Model file for the job. Use its own axes, mm. Face numbers are marked on the shaded views. A direction names the side the tool comes from. Coordinates: 2 decimals unless noted, no trailing zeros. Order: outer loops, then holes, each group sorted by start corner. A loop starts at its lowest first (then second) coordinate and runs counter-clockwise, first axis right, second up. Notation, with made-up numbers: (34.25, 34) -> (62.25, 34) arc R32 cw to (62.25, 64) -> close; hole circle Ø10 at (85.5, 39). An arc over 180 degrees is marked (long way). Use CSV: the item, a comma, the result in double quotes. Start each with the question number.
(1) Pin check, flat tips, straight feed: pin 1 Ø0.9 at (x, y) = (1.5, -11) entering from +Z; pin 2 Ø0.9 at (x, y) = (1.5, -7) entering from +Z; pin 3 Ø0.9 at (x, z) = (1.5, -21) entering from +Y. Stop position of each tip, or through.
(2) Pull direction Z, two halves, no side cores. Call the marked faces 1, 2, 3 and 4: pulls with the +Z half, pulls with the -Z half, needs draft (parallel to the pull), parting line crosses it, or undercut.
(3) Cut at D-D on y = 6.5. Write the cut outline in (x, z), plus the area to 3 significant figures.
(4) Tool access for the marked faces 5, 6 and 7: list every direction of +Z, -Z, +X, -X, +Y, -Y with a clear straight run to the whole face (end or side of a thin tool).
(5) Cut at B-B on x = 2.55. Write the cut outline in (y, z), plus the area to 3 significant figures.
(6) Cut at C-C on z = -1. Write the cut outline in (x, y).
(7) Probe L1, parallel to Z at x = 2.7, y = -9.5; L2, parallel to Z at x = 2, y = 8.75; L3, parallel to Y at x = 2.4, z = -18.5. List the from-to ranges inside material, lowest first.
(8) Cut at A-A on y = -10. Write the cut outline in (x, z).
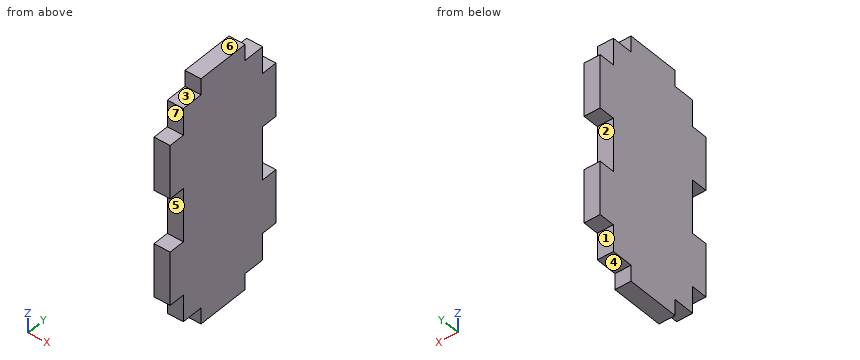
```python
from build123d import *

# Parameters (mm, degrees)
SKETCH1_W               = 46
SKETCH1_H               = 24
BOSS_EXTRUDE1_DEPTH     = 3
SKETCH2_W               = 5
SKETCH2_H               = 3
CUT_EXTRUDE1_DEPTH      = 4
MIRROR2_COPY_1_SKETCH_W = 5
MIRROR2_COPY_1_SKETCH_H = 3
MIRROR2_COPY_1_DEPTH    = 4


with BuildPart() as part:
    # Sketch1 → Boss-Extrude1 (new body)
    with BuildSketch(Plane(origin=(0, 0, 0), x_dir=(0, 0, -1), z_dir=(1, 0, 0))):
        Rectangle(SKETCH1_W, SKETCH1_H)
    extrude(amount=BOSS_EXTRUDE1_DEPTH)

    # Sketch2 → Cut-Extrude1 (cut, through all)
    with BuildSketch(Plane(origin=(3, 0, 0), x_dir=(0, 0, -1), z_dir=(1, 0, 0))):
        Polygon((23, 5), (20, 5), (20, 9), (15, 9), (15, 12), (23, 12), align=None)
        with Locations((2.5, 10.5)):
            Rectangle(SKETCH2_W, SKETCH2_H)
    cut_extrude1 = extrude(amount=-CUT_EXTRUDE1_DEPTH, mode=Mode.SUBTRACT)

    # Mirror1: Cut-Extrude1 across plane
    add(cut_extrude1.mirror(Plane.ZX), mode=Mode.SUBTRACT)

    # Mirror2: Cut-Extrude1 across plane
    add(cut_extrude1.mirror(Plane.XY), mode=Mode.SUBTRACT)

    # Mirror2 copy 1 sketch → Mirror2 copy 1 (cut, through all)
    with BuildSketch(Plane(origin=(3, 0, 0), x_dir=(0, 0, 1), z_dir=(1, 0, 0))):
        Polygon((23, 5), (20, 5), (20, 9), (15, 9), (15, 12), (23, 12), align=None)
        with Locations((2.5, 10.5)):
            Rectangle(MIRROR2_COPY_1_SKETCH_W, MIRROR2_COPY_1_SKETCH_H)
    extrude(amount=-MIRROR2_COPY_1_DEPTH, mode=Mode.SUBTRACT)


solid = part.part
```
Outcome:
1,pin 1,"z = 15"
1,pin 2,"z = 20"
1,pin 3,"y = 5"
2,face 1,"needs draft"
2,face 2,"undercut"
2,face 3,"pulls with the +Z half"
2,face 4,"pulls with the -Z half"
3,outline,"(0, -20) -> (3, -20) -> (3, 20) -> (0, 20) -> close"
3,area,"120 mm2"
4,face 5,"+X, -X, -Y"
4,face 6,"+Z, +X, -X, +Y, -Y"
4,face 7,"+Z, +X, -X, -Y"
5,outline,"(-12, -15) -> (-9, -15) -> (-9, -20) -> (-5, -20) -> (-5, -23) -> (5, -23) -> (5, -20) -> (9, -20) -> (9, -15) -> (12, -15) -> (12, -5) -> (9, -5) -> (9, 5) -> (12, 5) -> (12, 15) -> (9, 15) -> (9, 20) -> (5, 20) -> (5, 23) -> (-5, 23) -> (-5, 20) -> (-9, 20) -> (-9, 15) -> (-12, 15) -> (-12, 5) -> (-9, 5) -> (-9, -5) -> (-12, -5) -> close"
5,area,"900 mm2"
6,outline,"(0, -9) -> (3, -9) -> (3, 9) -> (0, 9) -> close"
7,L1,"-15 to -5, 5 to 15"
7,L2,"-20 to 20"
7,L3,"-9 to 9"
8,outline,"(0, -15) -> (3, -15) -> (3, -5) -> (0, -5) -> close; (0, 5) -> (3, 5) -> (3, 15) -> (0, 15) -> close"
